```python
from build123d import *

# Parameters (mm, degrees)
SKETCH_1_R          = 4.3
EXTRUDE_1_DEPTH     = 3
SKETCH_2_R          = 2.5
EXTRUDE_2_DEPTH     = 30
CUT_EXTRUDE_1_DEPTH = 1.5


with BuildPart() as part:
    # 草图1 → 凸台-拉伸1 (new body)
    with BuildSketch(Plane(origin=(0, 0, 0), x_dir=(1, 0, 0), z_dir=(0, 1, 0))):
        Circle(SKETCH_1_R)
    extrude(amount=EXTRUDE_1_DEPTH)

    # 草图2 → 凸台-拉伸2 (add)
    with BuildSketch(Plane(origin=(0, 3, 0), x_dir=(1, 0, 0), z_dir=(0, 1, 0))):
        Circle(SKETCH_2_R)
    extrude(amount=EXTRUDE_2_DEPTH)

    # 草图3 → 切除-拉伸1 (cut)
    with BuildSketch(Plane.XZ):
        with BuildLine():
            Line((-0.6, 1.1), (-0.6, 2.4))
            Line((-0.6, 2.4), (0.6, 2.4))
            Line((0.6, 2.4), (0.6, 1.1))
            ThreePointArc((0.6, 1.1), (0.746446609, 0.746446609), (1.1, 0.6))
            Line((1.1, 0.6), (2.4, 0.6))
            Line((2.4, 0.6), (2.4, -0.6))
            Line((2.4, -0.6), (1.1, -0.6))
            ThreePointArc((1.1, -0.6), (0.746446609, -0.746446609), (0.6, -1.1))
            Line((0.6, -1.1), (0.6, -2.4))
            Line((0.6, -2.4), (-0.6, -2.4))
            Line((-0.6, -2.4), (-0.6, -1.1))
            ThreePointArc((-0.6, -1.1), (-0.746446609, -0.746446609), (-1.1, -0.6))
            Line((-1.1, -0.6), (-2.4, -0.6))
            Line((-2.4, -0.6), (-2.4, 0.6))
            Line((-2.4, 0.6), (-1.1, 0.6))
            ThreePointArc((-1.1, 0.6), (-0.746446609, 0.746446609), (-0.6, 1.1))
        make_face()
    extrude(amount=-CUT_EXTRUDE_1_DEPTH, mode=Mode.SUBTRACT)


solid = part.part
```
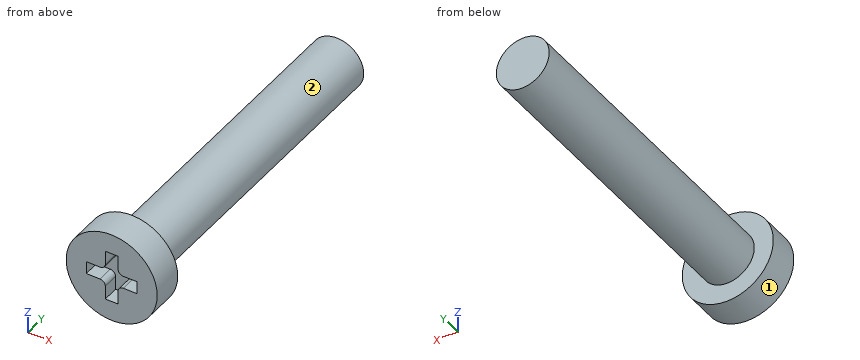
Read the model definition and answer for the solid it produces. Units are mm, in the model's axes. Face numbers are marked on the shaded views. A direction names the side the tool comes from. Give positions to 0.01 mm unless a question says otherwise; leave off trailing zeros. Loops run counter-clockwise (first coordinate to the right, second up) from the corner with the lowest first, then second, coordinate; pieces in that order, holes last.
Item 1: For the marked faces 1 and 2, determine the directions among +Z, -Z, +X, -X, +Y, -Y from which every point of the face is accessible in a straight line to the end or side of a thin tool.
Item 2: The part is cut by section B-B (x = 0). Write down the section's boundary in (y, z).
Item 3: The part is cut by section A-A (z = 0). Write down the section's boundary in (x, y).
Item 4: The part is cut by section D-D (x = -3). Write down the section's boundary in (y, z).
Item 5: The part is cut by section C-C (y = 25). Write down the section's boundary in (x, z), and give its area (3 significant figures).
Item 6: Each of these flat-tipped pins is pushed along its axis until it touches: pin 1 Ø0.6 at (x, y) = (-2, 0.5) entering from -Z; pin 2 Ø3 at (x, z) = (3.5, 2) entering from +Y; pin 3 Ø1.4 at (y, z) = (1, -2) entering from -X. Where does it stop, or does it pass through?
Item 7: Find the intervals of material crossed by line 1 along Y through (x, z) = (-2.5, 2.25); line 2 along Y through (x, z) = (-0.5, 0.5); line 3 along Z through (x, y) = (-0.5, 6), in increasing order.
Taken from the geometry:
1. face 1: +Y, -Y
1. face 2: +Y
2. outline: (0, -4.3) - (3, -4.3) - (3, -2.5) - (33, -2.5) - (33, 2.5) - (3, 2.5) - (3, 4.3) - (0, 4.3) - (0, 2.4) - (1.5, 2.4) - (1.5, -2.4) - (0, -2.4) - close
3. outline: (-4.3, 0) - (-2.4, 0) - (-2.4, 1.5) - (2.4, 1.5) - (2.4, 0) - (4.3, 0) - (4.3, 3) - (2.5, 3) - (2.5, 33) - (-2.5, 33) - (-2.5, 3) - (-4.3, 3) - close
4. outline: (0, -3.08) - (3, -3.08) - (3, 3.08) - (0, 3.08) - close
5. outline: circle Ø5 at (0, 0)
5. area: 19.6 mm2
6. pin 1: stops at z = -3.95
6. pin 2: stops at y = 3
6. pin 3: stops at x = -4.1
7. line 1: y = 0 to 3
7. line 2: y = 1.5 to 33
7. line 3: z = -2.45 to 2.45
